Model file for the job. Use its own axes, mm. A direction names the side the tool comes from. Coordinates: 2 decimals unless noted, no trailing zeros. Order: outer loops, then holes, each group sorted by start corner. A loop starts at its lowest first (then second) coordinate and runs counter-clockwise, first axis right, second up. Notation, with made-up numbers: (34, 29) -> (44, 29) arc R24 cw to (44, 57) -> close; hole circle Ø9 at (71, 50.5). An arc over 180 degrees is marked (long way). Write item = value, one per line. Start each with the question number.
Q1. Cut at B-B, the plane y = -3.75. List the corners of the cut face in (x, z), plus the area to 3 significant figures.
Q2. Cut at C-C, the plane z = 196. List the corners of the cut face in (x, y), plus the area to 3 significant figures.
Q3. 3-axis set-ups, long thin cutter, end or side, ignore diameter. For faces 4 (the face through (0.14, -11.41, 34.93)), 5 (the face through (0, -10.16, 113)): which of +Z, -Z, +X, -X, +Y, -Y reach the whole face in a straight line?
Q4. Cut at A-A, the plane z = 25.4. List the corners of the cut face in (x, y) (3 decimals).
Q5. Mould opens along Y. For faces 1 (the face through (0.95, 11.45, 28.43)), 2 (the face through (0, 12.7, 113)), 3 (the face through (0, 10.16, 113)) say: +Y half, -Y half, draft (parallel to the pull), parting line (faces both ways), or undercut.
Q6. Flat gauge pin, fed straight in: pin 1 (8 mm diameter, centred on x = 1.5, y = -4.5, fed in from -Z). Where does the tip first touch, or does it go through?
Q7. Cut at D-D, the plane x = 0. Give the number of separate pieces and of enclosed holes in the cut face, plus the area to 3 significant figures.
Q8. Wall check: line 1 (X direction, y = -5, z = 113); line 2 (X direction, y = -10.9, z = 203.2) (3 decimals). Give the ranges that are in metal, low to high. Write a range as from..to.
from build123d import *

# Parameters (mm, degrees)
SKETCH1_W           = 25.4
SKETCH1_H           = 25.4
SKETCH1_W_2         = 20.32
SKETCH1_H_2         = 20.32
BOSS_EXTRUDE2_DEPTH = 228.6
SKETCH3_R           = 3.175
CUT_EXTRUDE2_DEPTH  = 231.35713577


with BuildPart() as part:
    # Sketch1 → Boss-Extrude2 (new body)
    with BuildSketch(Plane.XY):
        Rectangle(SKETCH1_W, SKETCH1_H)
        Rectangle(SKETCH1_W_2, SKETCH1_H_2, mode=Mode.SUBTRACT)
    extrude(amount=BOSS_EXTRUDE2_DEPTH)

    # Sketch3 → Cut-Extrude2 (cut, through all)
    with BuildSketch(Plane(origin=(0, 12.7, 0), x_dir=(1, 0, 0), z_dir=(0, 1, 0))):
        with Locations(Location((0, -12.7, 0), (0, 0, 270))):
            Circle(SKETCH3_R)
        with Locations(Location((0, -25.4, 0), (0, 0, 270))):
            Circle(SKETCH3_R)
        with Locations(Location((0, -38.1, 0), (0, 0, 270))):
            Circle(SKETCH3_R)
        with Locations((0, -190.5)):
            Circle(SKETCH3_R)
        with Locations((0, -203.2)):
            Circle(SKETCH3_R)
        with Locations((0, -215.9)):
            Circle(SKETCH3_R)
    extrude(amount=-CUT_EXTRUDE2_DEPTH, mode=Mode.SUBTRACT)


solid = part.part
Here are the results:
q1.outline = (-12.7, 0) -> (-10.16, 0) -> (-10.16, 228.6) -> (-12.7, 228.6) -> close; (10.16, 0) -> (12.7, 0) -> (12.7, 228.6) -> (10.16, 228.6) -> close
q1.area = 1,160 mm²
q2.outline = (-12.7, -12.7) -> (12.7, -12.7) -> (12.7, 12.7) -> (-12.7, 12.7) -> close; hole (-10.16, -10.16) -> (10.16, -10.16) -> (10.16, 10.16) -> (-10.16, 10.16) -> close
q2.area = 232 mm²
q3.face_4 = +Y, -Y
q3.face_5 = +Z, -Z
q4.outline = (-12.7, -12.7) -> (-3.175, -12.7) -> (-3.175, -10.16) -> (-10.16, -10.16) -> (-10.16, 10.16) -> (-3.175, 10.16) -> (-3.175, 12.7) -> (-12.7, 12.7) -> close; (3.175, -12.7) -> (12.7, -12.7) -> (12.7, 12.7) -> (3.175, 12.7) -> (3.175, 10.16) -> (10.16, 10.16) -> (10.16, -10.16) -> (3.175, -10.16) -> close
q5.face_1 = draft
q5.face_2 = +Y half
q5.face_3 = undercut
q6.pin_1 = through
q7.separate_pieces = 14
q7.enclosed_holes = 0
q7.area = 968 mm²
q8.line_1 = -12.7..-10.16, 10.16..12.7
q8.line_2 = -12.7..-3.175, 3.175..12.7
